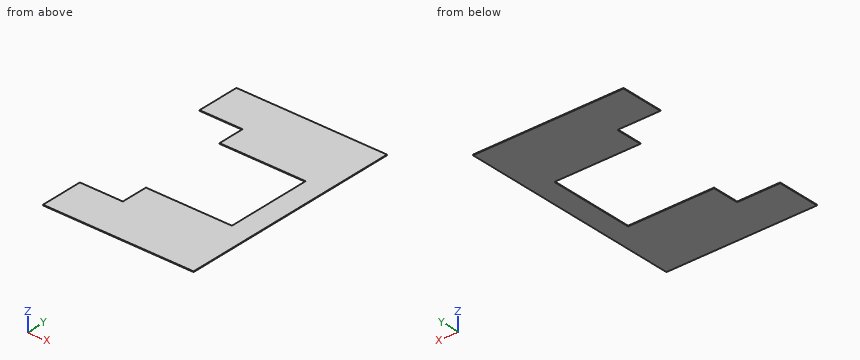
Autodesk Inventor part; units mm, degrees
ref_plane "YZ Plane" through (0, 0, 0) normal (1, 0, 0) x (0, 1, 0)
ref_plane "XZ Plane" through (0, 0, 0) normal (0, 1, 0) x (-1, 0, 0)
ref_plane "XY Plane" through (0, 0, 0) normal (0, 0, 1) x (1, 0, 0)
sketch "Sketch1" plane through (0, 0, 0) normal (0, 0, 1) x (1, 0, 0)
  line L0 (-355.6, 0) -> (-355.6, -101.6)
  line L1 (-355.6, -101.6) -> (0, -101.6)
  line L2 (0, -101.6) -> (0, 0)
  line L3 (-254, 330.2) -> (-355.6, 330.2)
  line L4 (-355.6, 330.2) -> (-355.6, 431.8)
  line L5 (-355.6, 431.8) -> (0, 431.8)
  line L6 (0, 0) -> (0, 431.8)
  line L7 (-355.6, 0) -> (-254, 0)
  line L8 (-254, 330.2) -> (-254, 266.7)
  line L9 (-254, 0) -> (-254, 63.5)
  line L10 (-254, 266.7) -> (-50.8, 266.7)
  line L11 (-50.8, 266.7) -> (-50.8, 63.5)
  line L12 (-50.8, 63.5) -> (-254, 63.5)
  dimension "d4" = 355.6
  dimension "d5" = 101.6
  dimension "d6" = 101.6
  dimension "d7" = 431.8
  dimension "d9" = 63.5
  dimension "d10" = 63.5
  dimension "d11" = 50.8
  dimension "d12" = 101.6
extrude "Extrusion1" add sketch "Sketch1" along normal blind 1.5875
properties part number "skid plate" material "Aluminum 6061"
Source: CAD feature listing. Evaluate the final solid. Frame: model axes, mm. Round coordinates to 2 decimals unless told otherwise and drop trailing zeros. Loops run counter-clockwise (first coordinate to the right, second up) from the corner with the lowest first, then second, coordinate; pieces in that order, holes last. Notation, with made-up numbers: (34, -16.5) - (56, -16.5) arc R20 ccw to (56, 9.5) - close; hole circle Ø11 at (12.5, 65.25). An arc over 180 degrees is marked (long way). Write item = value, one per line. Start each with the question number.
(1) Section query B-B, the plane z = 0.25. Output: boundary loops of the cut face in (x, y).
(2) Ray query, line 1 along Y through (x, z) = (-247, 1.45); line 2 along Y through (x, z) = (-297.5, 0.1); line 3 along X through (y, z) = (143.5, 0.7). Return the intervals inside material, ascending. Write a range as from..to.
(3) Pin query (flat end, axial travel): pin 1 (0.5 mm diameter, centred on y = 28, z = 1, fed in from -X). Return the tip coordinate at first contact, or that it passes through.
(4) Section query D-D, the plane y = 204. Output: boundary loops of the cut face in (x, z).
(5) Section query A-A, the plane x = -203.5. Output: boundary loops of the cut face in (y, z).
(6) Section query C-C, the plane x = -299.5. Output: boundary loops of the cut face in (y, z).
Conclusion:
q1.outline = (-355.6, -101.6) - (0, -101.6) - (0, 431.8) - (-355.6, 431.8) - (-355.6, 330.2) - (-254, 330.2) - (-254, 266.7) - (-50.8, 266.7) - (-50.8, 63.5) - (-254, 63.5) - (-254, 0) - (-355.6, 0) - close
q2.line_1 = -101.6..63.5, 266.7..431.8
q2.line_2 = -101.6..0, 330.2..431.8
q2.line_3 = -50.8..0
q3.pin_1 = -254
q4.outline = (-50.8, 0) - (0, 0) - (0, 1.59) - (-50.8, 1.59) - close
q5.outline = (-101.6, 0) - (63.5, 0) - (63.5, 1.59) - (-101.6, 1.59) - close; (266.7, 0) - (431.8, 0) - (431.8, 1.59) - (266.7, 1.59) - close
q6.outline = (-101.6, 0) - (0, 0) - (0, 1.59) - (-101.6, 1.59) - close; (330.2, 0) - (431.8, 0) - (431.8, 1.59) - (330.2, 1.59) - close
